Check sheet for the modelled part. Datum: model origin and axes. Units: mm. Face numbers are marked on the shaded views. A direction names the side the tool comes from. Give positions to 0.01 mm unless a question says otherwise; leave off trailing zeros. Loops run counter-clockwise (first coordinate to the right, second up) from the corner with the lowest first, then second, coordinate; pieces in that order, holes last. Notation, with made-up numbers: (28, 51) -> (74, 51) arc R24 ccw to (74, 88) -> close; hole circle Ø4 at (-32, -34). An arc over 180 degrees is marked (long way). Write each question's results on one line, items separated by ' | '. Start each with the question number.
1. Cross-section at B-B on y = 1.25. Record the boundary of the cut face in (x, z).
2. Cross-section at D-D on z = -15.5. Record the boundary of the cut face in (x, y), and give its area (3 significant figures).
3. Gauge pin test, flat ends, axial feed: pin 1 Ø4.5 at (x, z) = (30, -30) entering from +Y; pin 2 Ø11 at (x, z) = (11, -27.5) entering from +Y; pin 3 Ø8 at (x, z) = (30, -10) entering from +Y; pin 4 Ø5 at (x, y) = (35, 8) entering from -Z. Record the tip position at first contact, or that the pin passes through.
4. Material ranges on L1, parallel to X at y = 0.95, z = -30; L2, parallel to Z at x = 10, y = 1.35; L3, parallel to Z at x = 9, y = 4, recorded low to high. Write a range as from..to.
5. Cross-section at A-A on z = -30. Count the separate pieces of the cut face and the enclosed holes in it, and give its area (3 significant figures).
6. Tool access check on the marked faces 4 and 5. Record the directions out of +Z, -Z, +X, -X, +Y, -Y that give a thin tool (end or side, any length) a straight path to the whole face; none if there is none.
7. Mould release check, pull along Z, two halves, no side actions. Record for the marked faces 1, 2 and 3: +Z half, -Z half, draft (parallel to the pull), parting line (faces both ways), or undercut.
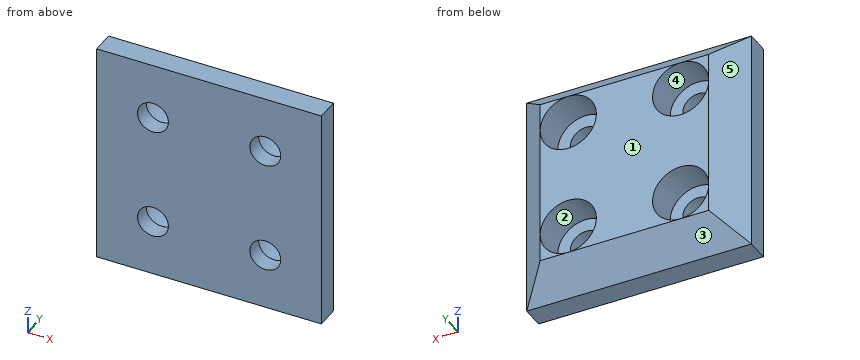
from build123d import *

# Parameters (mm, degrees)
SKETCH1_W           = 40
SKETCH1_H           = 40
SKETCH1_R           = 2.75
BOSS_EXTRUDE1_DEPTH = 9
SKETCH2_R           = 5
CUT_EXTRUDE1_DEPTH  = 6
CHAMFER1_SIZE       = 5


with BuildPart() as part:
    # Sketch1 → Boss-Extrude1 (new body)
    with BuildSketch(Plane(origin=(0, 0, 0), x_dir=(1, 0, 0), z_dir=(0, 1, 0))):
        with Locations((20, 20)):
            Rectangle(SKETCH1_W, SKETCH1_H)
        with Locations(Location((10, 30, 0), (0, 0, 270))):
            Circle(SKETCH1_R, mode=Mode.SUBTRACT)
        with Locations(Location((30, 30, 0), (0, 0, 270))):
            Circle(SKETCH1_R, mode=Mode.SUBTRACT)
        with Locations(Location((30, 10, 0), (0, 0, 270))):
            Circle(SKETCH1_R, mode=Mode.SUBTRACT)
        with Locations(Location((10, 10, 0), (0, 0, 270))):
            Circle(SKETCH1_R, mode=Mode.SUBTRACT)
    extrude(amount=BOSS_EXTRUDE1_DEPTH)

    # Sketch2 → Cut-Extrude1 (cut)
    with BuildSketch(Plane(origin=(0, 9, 0), x_dir=(1, 0, 0), z_dir=(0, 1, 0))):
        with Locations(Location((10, 10, 0), (0, 0, 270))):
            Circle(SKETCH2_R)
        with Locations(Location((30, 10, 0), (0, 0, 270))):
            Circle(SKETCH2_R)
        with Locations(Location((30, 30, 0), (0, 0, 270))):
            Circle(SKETCH2_R)
        with Locations(Location((10, 30, 0), (0, 0, 270))):
            Circle(SKETCH2_R)
    extrude(amount=-CUT_EXTRUDE1_DEPTH, mode=Mode.SUBTRACT)

    # Chamfer1
    chamfer1_edges = [part.edges().sort_by_distance(p)[0] for p in [
        (40, 9, -20),
        (20, 9, -40),
        (0, 9, -20),
        (20, 9, 0),
    ]]
    chamfer(chamfer1_edges, length=CHAMFER1_SIZE - 0.0001)  # a hair under: the kernel refuses the full size


solid = part.part
Geometry says:
1) outline: (0, -40) -> (40, -40) -> (40, 0) -> (0, 0) -> close; hole circle Ø5.5 at (10, -30); hole circle Ø5.5 at (10, -10); hole circle Ø5.5 at (30, -30); hole circle Ø5.5 at (30, -10)
2) outline: (0, 0) -> (40, 0) -> (40, 4) -> (35, 9) -> (5, 9) -> (0, 4) -> close | area: 335 mm^2
3) pin 1: through | pin 2: y = 9 | pin 3: y = 3 | pin 4: z = -38.5
4) L1: 0..7.25, 12.75..27.25, 32.75..40 | L2: -40..-32.75, -27.25..-12.75, -7.25..0 | L3: -40..-34.9, -25.1..-14.9, -5.1..0
5) separate pieces: 3 | enclosed holes: 0 | area: 182 mm^2
6) face 4: +Y | face 5: +Z, -Z, -X, +Y
7) face 1: draft | face 2: undercut | face 3: -Z half
